```python
from build123d import *

# Parameters (mm, degrees)
F1_DEPTH = 3.81
F0_R     = 3.175
F2_DEPTH = 3.81


# Not quite as in the source:
# - a feature names something its author has since deleted; it is built from what else it names


with BuildPart() as f1:
    # F0 (on Top) → F1 (new body)
    with BuildSketch(Plane.XY):
        with BuildLine():
            ThreePointArc((-3.175, 52.07), (0, 55.245), (3.175, 52.07))
            Line((3.175, 52.07), (6.35, 52.07))
            ThreePointArc((6.35, 52.07), (0, 58.42), (-6.35, 52.07))
            Line((-6.35, 52.07), (-3.175, 52.07))
        make_face()
    extrude(amount=F1_DEPTH)

    # F0 (on Top) → F2 (join)
    with BuildSketch(Plane.XY):
        Polygon((0, -52.07), (6.35, -34.2291146517), (-6.35, -34.2291146517), align=None)
        with BuildLine():
            Line((6.35, 52.07), (3.175, 52.07))
            ThreePointArc((3.175, 52.07), (0, 48.895), (-3.175, 52.07))
            Line((-3.175, 52.07), (-6.35, 52.07))
            Line((-6.35, 52.07), (-6.35, -34.2291146517))
            Line((-6.35, -34.2291146517), (6.35, -34.2291146517))
            Line((6.35, -34.2291146517), (6.35, 52.07))
        make_face()
        with Locations((0, -12.192)):
            Circle(F0_R, mode=Mode.SUBTRACT)
    extrude(amount=F2_DEPTH)


solid = f1.part
```
Source: CAD feature listing. Evaluate the final solid. Frame: model axes, mm. Round coordinates to 2 decimals unless told otherwise and drop trailing zeros. Loops run counter-clockwise (first coordinate to the right, second up) from the corner with the lowest first, then second, coordinate; pieces in that order, holes last. Notation, with made-up numbers: M 30,16.25 L 52,16.25 A24 ccw 52,37.25 Z; hole C 2,0 d1. An arc over 180 degrees is marked long. Use a Markdown table: item, result. Add a question column.
1. Section query A-A on x = 1.75. Return the cut outline in (y, z), then the cut area to 3 significant figures.
2. Contact query for a flat-ended pin moving along its axis: P1, Ø2, axis at x = 4.5, z = 3.5, coming from the +Y side. Output: stop coordinate, or through.
3. Section query B-B on z = 2.6. Return the cut outline in (x, y) (3 decimals).
4. Mould query, pull axis X, two halves, no side actions, for faces 1 (the cylindrical face through (-0.413, -9.044, 1.878)), 2 (the flat face through (6.35, 8, 2)), 3 (the flat face through (-6.35, 10, 2)). Classes: pulls with the +X half, pulls with the -X half, needs draft (parallel to the pull), parting line crosses it, or undercut.
5. Line query: line 1 (X direction, y = 52.07, z = 1.85) (3 decimals); line 2 (X direction, y = 50.5, z = 1.75); line 3 (X direction, y = -43.5, z = 3.6). Output: solid intervals per line, ascending.
Reported:
| question | item | result |
|---|---|---|
| 1 | outline | M -47.15,0 L -14.84,0 L -14.84,3.81 L -47.15,3.81 Z; M -9.54,0 L 49.42,0 L 49.42,3.81 L -9.54,3.81 Z; M 54.72,0 L 58.17,0 L 58.17,3.81 L 54.72,3.81 Z |
| 1 | area | 361 mm² |
| 2 | P1 | stops at y = 57.37 |
| 3 | outline | M -6.35,-34.229 L 0,-52.07 L 6.35,-34.229 L 6.35,52.07 A6.35 ccw -6.35,52.07 Z; hole C 0,-12.192 d6.35; hole C 0,52.07 d6.35 |
| 4 | face 1 | undercut |
| 4 | face 2 | pulls with the +X half |
| 4 | face 3 | pulls with the -X half |
| 5 | line 1 | x = -6.35 to -3.175, 3.175 to 6.35 |
| 5 | line 2 | x = -6.35 to -2.76, 2.76 to 6.35 |
| 5 | line 3 | x = -3.05 to 3.05 |
